from build123d import *

# Parameters (mm, degrees)
F1_DEPTH = 10
F3_D     = 10
F3_DEPTH = 12


with BuildPart() as f1:
    # F0 (on Front) → F1 (new body, symmetric)
    with BuildSketch(Plane.XZ):
        with BuildLine():
            Line((10, 0), (-10, 0))
            Line((-10, 0), (-10, -6))
            Line((-10, -6), (15, -6))
            Line((15, -6), (15, 14))
            ThreePointArc((15, 14), (16.171573, 16.828427), (19, 18))
            Line((19, 18), (25, 18))
            Line((25, 18), (25, 23))
            Line((25, 23), (18, 23))
            ThreePointArc((18, 23), (12.343146, 20.656854), (10, 15))
            Line((10, 15), (10, 0))
        make_face()
    extrude(amount=F1_DEPTH, both=True)

    # F3
    with Locations(Plane.XY):
        with Locations((0, 0)):
            Hole(F3_D / 2, depth=F3_DEPTH)


solid = f1.part
Check sheet for the modelled part. Datum: model origin and axes. Units: mm. A direction names the side the tool comes from. Give positions to 0.01 mm unless a question says otherwise; leave off trailing zeros. Write each loop counter-clockwise with the first axis right and the second up, starting at its lowest first coordinate (ties: lowest second). Pieces come first, ordered by that corner, then holes. Notation, with made-up numbers: M -15.75,68.5 L 40.25,68.5 A17 ccw 40.25,73.5 Z; hole C 39,-23.5 d9. An arc over 180 degrees is marked long. Use one line per item in the form item = value.
(1) Section check B-B on y = 0. Record the boundary of the cut face in (x, z), plus the area to 3 significant figures.
Answer block:
outline = M -10,-6 L -5,-6 L -5,0 L -10,0 Z; M 5,-6 L 15,-6 L 15,14 A4 cw 19,18 L 25,18 L 25,23 L 18,23 A8 ccw 10,15 L 10,0 L 5,0 Z
area = 245 mm2
(2) Section check A-A on x = 0. Record the boundary of the cut face in (y, z).
Answer block:
outline = M -10,-6 L -5,-6 L -5,0 L -10,0 Z; M 5,-6 L 10,-6 L 10,0 L 5,0 Z
(3) Depth check by flat-ended pin: P1, Ø3, axis at x = 20.5, y = 0.5, coming from the -Z side; P2, Ø6, axis at y = -1, z = 14.5, coming from the -X side; P3, Ø11.5, axis at x = 0, y = 0, coming from the +Z side. Enter the tip coordinate at first touch or a pass-through.
Answer block:
P1 = 18
P2 = 10
P3 = 0
(4) Section check C-C on y = -6. Record the boundary of the cut face in (x, z), plus the area to 3 significant figures.
Answer block:
outline = M -10,-6 L 15,-6 L 15,14 A4 cw 19,18 L 25,18 L 25,23 L 18,23 A8 ccw 10,15 L 10,0 L -10,0 Z
area = 305 mm2
(5) Tool access check on faces 4 (the flat face through (2, -5, 0)), 5 (the flat face through (25, 0, 20)), 6 (the flat face through (15, 0, 4)). Record the directions out of +Z, -Z, +X, -X, +Y, -Y that give a thin tool (end or side, any length) a straight path to the whole face; none if there is none.
Answer block:
face_4 = +Z, -X, +Y, -Y
face_5 = +Z, -Z, +X, +Y, -Y
face_6 = -Z, +X, +Y, -Y
(6) Section check D-D on z = 2.25. Record the boundary of the cut face in (x, y).
Answer block:
outline = M 10,-10 L 15,-10 L 15,10 L 10,10 Z
(7) Draft check along Y on faces 1 (the flat face through (22, 0, 18)), 2 (the flat face through (11, -10, 6)), 3 (the cylindrical face through (1.08, -4.88, -3.04)). Enter one of: pulls with the +Y half, pulls with the -Y half, needs draft (parallel to the pull), parting line crosses it, or undercut.
Answer block:
face_1 = needs draft
face_2 = pulls with the -Y half
face_3 = undercut
(8) Material ranges on line 1 along Y through (x, z) = (0, -4.45); line 2 along Z through (x, y) = (9, 6.75); line 3 along Z through (x, y) = (21.5, -3.25), recorded low to high.
Answer block:
line_1 = -10 to -5, 5 to 10
line_2 = -6 to 0
line_3 = 18 to 23
